The listing builds one solid part. Answer for the finished solid, in the listing's coordinates (mm). Face numbers are marked on the shaded views. A direction names the side the tool comes from. Give positions to 0.01 mm unless a question says otherwise; leave off trailing zeros. Order: outer loops, then holes, each group sorted by start corner. A loop starts at its lowest first (then second) coordinate and runs counter-clockwise, first axis right, second up. Notation, with made-up numbers: (74.5, -29.75) - (103.5, -29.75) arc R16 ccw to (103.5, -9.75) - close; hole circle Ø2 at (70, 70.25). An arc over 180 degrees is marked (long way). Write each question's results on one line, items separated by ' | '. Start each with the question number.
1. Find the intervals of material crossed by L1, parallel to Y at x = 101, z = 1250; L2, parallel to Y at x = 0, z = 62; L3, parallel to Z at x = 352, y = 590, in increasing order.
2. Section D-D (x = 424) is taken. Give the vertices of the cut face in (y, z).
3. Section A-A (y = 0) is taken. Give the vertices of the cut face in (x, z), and give its area (3 significant figures).
4. Which of the six approach directions +Z, -Z, +X, -X, +Y, -Y give full straight-line access (tool end or side, diameter ignored) to the marked faces 1, 2, 3 and 4?
5. Section C-C (y = 454) is taken. Give the vertices of the cut face in (x, z).
6. Flat-ended cylindrical pins translate along their axes: pin 1 (1.5 mm diameter, centred on y = -380.5, z = 919.5, fed in from +X); pin 2 (12 mm diameter, centred on y = -411, z = 917, fed in from -X); pin 3 (12 mm diameter, centred on x = -58.5, z = 770, fed in from -Y). Find the tip coordinate at first contact, or state that the pin passes through.
7. Section B-B (x = 0) is taken. Give the vertices of the cut face in (y, z).
8. Determine the mould class of the marked faces 5, 6 and 7 for opening direction Y: released by +Y, released by -Y, zero draft, split by the parting line, or undercut.
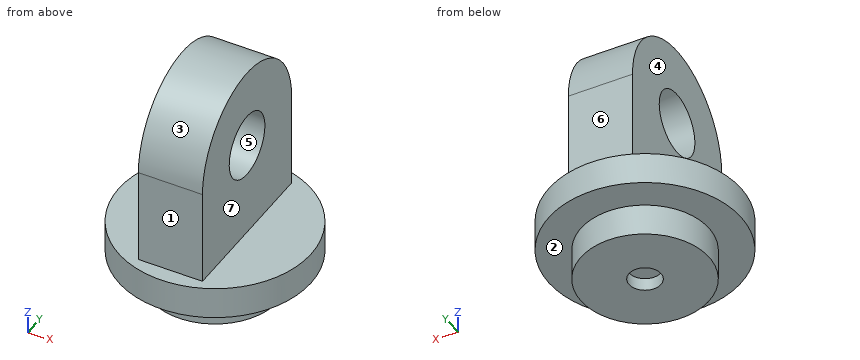
from build123d import *

# Parameters (mm, degrees)
SKETCH1_R           = 500
BOSS_EXTRUDE1_DEPTH = 250
SKETCH3_R           = 125
CUT_EXTRUDE1_DEPTH  = 100
SKETCH4_R           = 750
BOSS_EXTRUDE2_DEPTH = 250
SKETCH5_R           = 250
BOSS_EXTRUDE4_DEPTH = 250


with BuildPart() as part:
    # Sketch1 → Boss-Extrude1 (new body)
    with BuildSketch(Plane.XY):
        Circle(SKETCH1_R)
    extrude(amount=BOSS_EXTRUDE1_DEPTH)

    # Sketch3 → Cut-Extrude1 (cut)
    with BuildSketch(Plane(origin=(0, 0, 0), x_dir=(-1, 0, 0), z_dir=(0, 0, -1))):
        Circle(SKETCH3_R)
    extrude(amount=-CUT_EXTRUDE1_DEPTH, mode=Mode.SUBTRACT)

    # Sketch4 → Boss-Extrude2 (add)
    with BuildSketch(Plane.XY.offset(250)):
        Circle(SKETCH4_R)
    extrude(amount=BOSS_EXTRUDE2_DEPTH)

    # Sketch5 → Boss-Extrude4 (add, symmetric)
    with BuildSketch(Plane(origin=(0, 0, 0), x_dir=(0, 0, -1), z_dir=(1, 0, 0))):
        with BuildLine():
            Line((-1250, 625), (-500, 625))
            Line((-500, 625), (-500, -625))
            Line((-500, -625), (-1250, -625))
            ThreePointArc((-1250, -625), (-1875, 0), (-1250, 625))
        make_face()
        with Locations((-1250, 0)):
            Circle(SKETCH5_R, mode=Mode.SUBTRACT)
    extrude(amount=BOSS_EXTRUDE4_DEPTH, both=True)


solid = part.part
Reported:
1) L1: -625 to -250, 250 to 625 | L2: -500 to -125, 125 to 500 | L3: 250 to 500
2) outline: (-618.65, 250) - (-265, 250) - (-265, 0) - (265, 0) - (265, 250) - (618.65, 250) - (618.65, 500) - (-618.65, 500) - close
3) outline: (-750, 250) - (-500, 250) - (-500, 0) - (-125, 0) - (-125, 100) - (125, 100) - (125, 0) - (500, 0) - (500, 250) - (750, 250) - (750, 500) - (250, 500) - (250, 1000) - (-250, 1000) - (-250, 500) - (-750, 500) - close; (-250, 1500) - (250, 1500) - (250, 1875) - (-250, 1875) - close | area: 1,040,000 mm²
4) face 1: +Z, +X, -X, -Y | face 2: -Z | face 3: +Z, +X, -X | face 4: +Z, -X, +Y, -Y
5) outline: (-596.98, 250) - (-209.49, 250) - (-209.49, 0) - (209.49, 0) - (209.49, 250) - (596.98, 250) - (596.98, 500) - (250, 500) - (250, 1679.55) - (-250, 1679.55) - (-250, 500) - (-596.98, 500) - close
6) pin 1: x = 250 | pin 2: x = -250 | pin 3: y = -625
7) outline: (-750, 250) - (-500, 250) - (-500, 0) - (-125, 0) - (-125, 100) - (125, 100) - (125, 0) - (500, 0) - (500, 250) - (750, 250) - (750, 500) - (625, 500) - (625, 1250) arc R625 ccw to (-625, 1250) - (-625, 500) - (-750, 500) - close; hole circle Ø500 at (0, 1250)
8) face 5: undercut | face 6: released by +Y | face 7: zero draft
